```python
from build123d import *

# Parameters (mm, degrees)
SKETCH1_R           = 47.116713319
BOSS_EXTRUDE1_DEPTH = 3


with BuildPart() as part:
    # Sketch1 → Boss-Extrude1 (new body)
    with BuildSketch(Plane(origin=(0, 0, 0), x_dir=(1, 0, 0), z_dir=(0, 1, 0))):
        Polygon((-88.068159647, -47.370869281), (-99.999999495, 0.010045682), (-99.954698159, 3.009703627), (-86.597517101, 50.008699563), (-85.05845602, 52.583828878), (-49.991299932, 86.607562782), (-47.370869281, 88.068159647), (0.010045682, 99.999999495), (3.009703627, 99.954698159), (50.008699563, 86.597517101), (52.583828878, 85.05845602), (86.607562782, 49.991299932), (88.068159647, 47.370869281), (99.999999495, -0.010045682), (99.954698159, -3.009703627), (86.597517101, -50.008699563), (85.05845602, -52.583828878), (49.991299932, -86.607562782), (47.370869281, -88.068159647), (-0.010045682, -99.999999495), (-3.009703627, -99.954698159), (-50.008699563, -86.597517101), (-52.583828878, -85.05845602), (-86.607562782, -49.991299932), align=None)
        with Locations(Location((0, 0, 0), (0, 0, 270))):
            Circle(SKETCH1_R, mode=Mode.SUBTRACT)
    extrude(amount=BOSS_EXTRUDE1_DEPTH)


solid = part.part
```
The model under review builds one solid part; all positions refer to its coordinate system, in mm. Coordinates: 2 decimals unless noted, no trailing zeros. Write each loop counter-clockwise with the first axis right and the second up, starting at its lowest first coordinate (ties: lowest second). Pieces come first, ordered by that corner, then holes. Notation, with made-up numbers: (54, 34.25) - (111, 34.25) arc R28 ccw to (111, 70.25) - close; hole circle Ø9 at (43, 19.25). An arc over 180 degrees is marked (long way). Answer in a Markdown table with one row per item. Add a question column.
Q1. Consider section D-D on z = 71.5. Give the boundary of the cut face in (x, y).
Q2. To check wall thickness, follow line 1 along X through (y, z) = (1.7, 0); line 2 along Z through (x, y) = (20, 0.1). State the ranges of each line that lie inside material, in increasing order. Write a range as from..to.
Q3. Consider section C-C on z = 25.5. Give the boundary of the cut face in (x, y).
Q4. Draft analysis for pull direction Z (two halves, no side actions). For faces 1 (the face through (-43, 0, 21)), 2 (the face through (-28.67, 1.48, -37.39)), 3 (the face through (26.18, 1.48, -93.37)), state which applies: +Z half, -Z half, draft (parallel to the pull), parting line (faces both ways), or undercut.
Q5. Consider section B-B on x = 12.5. Give the boundary of the cut face in (y, z).
Q6. Consider section A-A on y = 1.55. Give the boundary of the cut face in (x, z).
Q7. Clearance check with flat-ended pins moving along their axes: pin 1 (1.5 mm diameter, centred on x = 11.5, y = 1, fed in from +Z); pin 2 (1 mm diameter, centred on x = -38.5, y = 2.5, fed in from -Z). State where each tip first meets the part, or that it passes through.
Answers below:
| question | item | result |
|---|---|---|
| 1 | outline | (-65.74, 0) - (65.56, 0) - (65.56, 3) - (-65.74, 3) - close |
| 2 | line 1 | -100..-47.12, 47.12..100 |
| 2 | line 2 | -95.13..-42.66, 42.66..94.96 |
| 3 | outline | (-93.58, 0) - (-39.62, 0) - (-39.62, 3) - (-93.58, 3) - close; (39.62, 0) - (93.56, 0) - (93.56, 3) - (39.62, 3) - close |
| 4 | face 1 | draft |
| 4 | face 2 | undercut |
| 4 | face 3 | -Z half |
| 5 | outline | (0, -97.26) - (3, -97.26) - (3, -45.43) - (0, -45.43) - close; (0, 45.43) - (3, 45.43) - (3, 96.85) - (0, 96.85) - close |
| 6 | outline | (-100, -0.01) - (-99.95, -3.01) - (-86.6, -50.01) - (-85.06, -52.58) - (-49.99, -86.61) - (-47.37, -88.07) - (0.01, -100) - (3.01, -99.95) - (50.01, -86.6) - (52.58, -85.06) - (86.61, -49.99) - (88.07, -47.37) - (100, 0.01) - (99.95, 3.01) - (86.6, 50.01) - (85.06, 52.58) - (49.99, 86.61) - (47.37, 88.07) - (-0.01, 100) - (-3.01, 99.95) - (-50.01, 86.6) - (-52.58, 85.06) - (-86.61, 49.99) - (-88.07, 47.37) - close; hole circle Ø94.23 at (0, 0) |
| 7 | pin 1 | z = 97.29 |
| 7 | pin 2 | z = -90.43 |
